from build123d import *

# Parameters (mm, degrees)
F2_DEPTH = 545


with BuildPart() as f2:
    # F0 (on Front) → F2 (new body)
    with BuildSketch(Plane.XZ):
        with BuildLine():
            Line((5.0927712857, 0), (1.5, 0))
            ThreePointArc((1.5, 0), (0.4393398282, -0.4393398282), (0, -1.5))
            Line((0, -1.5), (0, -5.0927712857))
            ThreePointArc((0, -5.0927712857), (0.0601351693, -5.3950911973), (0.2313856429, -5.6513856429))
            Line((0.2313856429, -5.6513856429), (1.69, -7.11))
            Line((1.69, -7.11), (1.8, -7.11))
            Line((1.8, -7.11), (1.8, -4.5006601718))
            Line((1.8, -4.5006601718), (3.44, -4.5006601718))
            Line((3.44, -4.5006601718), (6.1000000155, -7.1606601718))
            Line((6.1000000155, -7.1606601718), (6.1000000155, -9.9))
            Line((6.1000000155, -9.9), (6.2000000155, -10))
            Line((6.2000000155, -10), (6.1000000155, -10.1))
            Line((6.1000000155, -10.1), (6.1000000155, -12.8393398605))
            Line((6.1000000155, -12.8393398605), (3.44, -15.4993398916))
            Line((3.44, -15.4993398916), (1.8, -15.4993398916))
            Line((1.8, -15.4993398916), (1.8, -12.8893398916))
            Line((1.8, -12.8893398916), (1.69, -12.8893398916))
            Line((1.69, -12.8893398916), (0.2313856429, -14.3479542487))
            ThreePointArc((0.2313856429, -14.3479542487), (0.0601351693, -14.6042486943), (0, -14.9065686059))
            Line((0, -14.9065686059), (0, -20))
            Line((0, -20), (0, -25.0934313941))
            ThreePointArc((0, -25.0934313941), (0.0601351693, -25.3957513057), (0.2313856429, -25.6520457513))
            Line((0.2313856429, -25.6520457513), (1.69, -27.1106601084))
            Line((1.69, -27.1106601084), (1.8, -27.1106601084))
            Line((1.8, -27.1106601084), (1.8, -24.5006601084))
            Line((1.8, -24.5006601084), (3.44, -24.5006601084))
            Line((3.44, -24.5006601084), (6.1000000155, -27.1606601395))
            Line((6.1000000155, -27.1606601395), (6.1000000155, -29.9))
            Line((6.1000000155, -29.9), (6.2000000155, -30))
            Line((6.2000000155, -30), (6.1000000155, -30.1))
            Line((6.1000000155, -30.1), (6.1000000155, -32.8393398282))
            Line((6.1000000155, -32.8393398282), (3.44, -35.4993398282))
            Line((3.44, -35.4993398282), (1.8, -35.4993398282))
            Line((1.8, -35.4993398282), (1.8, -32.89))
            Line((1.8, -32.89), (1.69, -32.89))
            Line((1.69, -32.89), (0.2313856429, -34.3486143571))
            ThreePointArc((0.2313856429, -34.3486143571), (0.0601351693, -34.6049088027), (0, -34.9072287143))
            Line((0, -34.9072287143), (0, -38.5))
            ThreePointArc((0, -38.5), (0.4393398282, -39.5606601718), (1.5, -40))
            Line((1.5, -40), (5.0927712857, -40))
            ThreePointArc((5.0927712857, -40), (5.3950911973, -39.9398648307), (5.6513856429, -39.7686143571))
            Line((5.6513856429, -39.7686143571), (7.11, -38.31))
            Line((7.11, -38.31), (7.11, -38.2))
            Line((7.11, -38.2), (4.5006601718, -38.2))
            Line((4.5006601718, -38.2), (4.5006601718, -36.56))
            Line((4.5006601718, -36.56), (7.1606601873, -33.9))
            Line((7.1606601873, -33.9), (9.9000000155, -33.9))
            Line((9.9000000155, -33.9), (10.0000000478, -33.8000000323))
            Line((10.0000000478, -33.8000000323), (10.1000000802, -33.9))
            Line((10.1000000802, -33.9), (12.8393399084, -33.9))
            Line((12.8393399084, -33.9), (15.4993399239, -36.56))
            Line((15.4993399239, -36.56), (15.4993399239, -38.2))
            Line((15.4993399239, -38.2), (12.8900000957, -38.2))
            Line((12.8900000957, -38.2), (12.8900000957, -38.31))
            Line((12.8900000957, -38.31), (14.3486144528, -39.7686143571))
            ThreePointArc((14.3486144528, -39.7686143571), (14.6049088984, -39.9398648307), (14.90722881, -40))
            Line((14.90722881, -40), (18.5000000957, -40))
            ThreePointArc((18.5000000957, -40), (19.5606602675, -39.5606601718), (20.0000000957, -38.5))
            Line((20.0000000957, -38.5), (20.0000000957, -34.9072287143))
            ThreePointArc((20.0000000957, -34.9072287143), (19.9398649264, -34.6049088027), (19.7686144528, -34.3486143571))
            Line((19.7686144528, -34.3486143571), (18.3100000957, -32.89))
            Line((18.3100000957, -32.89), (18.2000000957, -32.89))
            Line((18.2000000957, -32.89), (18.2000000957, -35.4993398282))
            Line((18.2000000957, -35.4993398282), (16.5600000957, -35.4993398282))
            Line((16.5600000957, -35.4993398282), (13.9000000802, -32.8393398282))
            Line((13.9000000802, -32.8393398282), (13.9000000802, -30.1))
            Line((13.9000000802, -30.1), (13.8000000802, -30))
            Line((13.8000000802, -30), (13.9000000802, -29.9))
            Line((13.9000000802, -29.9), (13.9000000802, -27.1606601395))
            Line((13.9000000802, -27.1606601395), (16.5600000957, -24.5006601084))
            Line((16.5600000957, -24.5006601084), (18.2000000957, -24.5006601084))
            Line((18.2000000957, -24.5006601084), (18.2000000957, -27.1106601084))
            Line((18.2000000957, -27.1106601084), (18.3100000957, -27.1106601084))
            Line((18.3100000957, -27.1106601084), (19.7686144528, -25.6520457513))
            ThreePointArc((19.7686144528, -25.6520457513), (19.9398649264, -25.3957513057), (20.0000000957, -25.0934313941))
            Line((20.0000000957, -25.0934313941), (20.0000000957, -20))
            Line((20.0000000957, -20), (20.0000000957, -14.9065686059))
            ThreePointArc((20.0000000957, -14.9065686059), (19.9398649264, -14.6042486943), (19.7686144528, -14.3479542487))
            Line((19.7686144528, -14.3479542487), (18.3100000957, -12.8893398916))
            Line((18.3100000957, -12.8893398916), (18.2000000957, -12.8893398916))
            Line((18.2000000957, -12.8893398916), (18.2000000957, -15.4993398916))
            Line((18.2000000957, -15.4993398916), (16.5600000957, -15.4993398916))
            Line((16.5600000957, -15.4993398916), (13.9000000802, -12.8393398605))
            Line((13.9000000802, -12.8393398605), (13.9000000802, -10.1))
            Line((13.9000000802, -10.1), (13.8000000802, -10))
            Line((13.8000000802, -10), (13.9000000802, -9.9))
            Line((13.9000000802, -9.9), (13.9000000802, -7.1606601718))
            Line((13.9000000802, -7.1606601718), (16.5600000957, -4.5006601718))
            Line((16.5600000957, -4.5006601718), (18.2000000957, -4.5006601718))
            Line((18.2000000957, -4.5006601718), (18.2000000957, -7.11))
            Line((18.2000000957, -7.11), (18.3100000957, -7.11))
            Line((18.3100000957, -7.11), (19.7686144528, -5.6513856429))
            ThreePointArc((19.7686144528, -5.6513856429), (19.9398649264, -5.3950911973), (20.0000000957, -5.0927712857))
            Line((20.0000000957, -5.0927712857), (20.0000000957, -1.5))
            ThreePointArc((20.0000000957, -1.5), (19.5606602675, -0.4393398282), (18.5000000957, 0))
            Line((18.5000000957, 0), (14.90722881, 0))
            ThreePointArc((14.90722881, 0), (14.6049088984, -0.0601351693), (14.3486144528, -0.2313856429))
            Line((14.3486144528, -0.2313856429), (12.8900000957, -1.69))
            Line((12.8900000957, -1.69), (12.8900000957, -1.8))
            Line((12.8900000957, -1.8), (15.4993399239, -1.8))
            Line((15.4993399239, -1.8), (15.4993399239, -3.44))
            Line((15.4993399239, -3.44), (12.8393399084, -6.1))
            Line((12.8393399084, -6.1), (10.1000000802, -6.1))
            Line((10.1000000802, -6.1), (10.0000000478, -6.1999999677))
            Line((10.0000000478, -6.1999999677), (9.9000000155, -6.1))
            Line((9.9000000155, -6.1), (7.1606601873, -6.1))
            Line((7.1606601873, -6.1), (4.5006601718, -3.44))
            Line((4.5006601718, -3.44), (4.5006601718, -1.8))
            Line((4.5006601718, -1.8), (7.11, -1.8))
            Line((7.11, -1.8), (7.11, -1.69))
            Line((7.11, -1.69), (5.6513856429, -0.2313856429))
            ThreePointArc((5.6513856429, -0.2313856429), (5.3950911973, -0.0601351693), (5.0927712857, 0))
        make_face()
        Polygon((1.8, -38.2), (1.8, -36.57), (2.34, -36.57), (3.43, -37.66), (3.43, -38.2), align=None, mode=Mode.SUBTRACT)
        with BuildLine():
            ThreePointArc((10.0000000478, -27.9), (11.4849242883, -28.5150757595), (12.1000000478, -30))
            ThreePointArc((12.1000000478, -30), (11.4849242883, -31.4849242405), (10.0000000478, -32.1))
            ThreePointArc((10.0000000478, -32.1), (8.5150758074, -31.4849242405), (7.9000000478, -30))
            ThreePointArc((7.9000000478, -30), (8.5150758074, -28.5150757595), (10.0000000478, -27.9))
        make_face(mode=Mode.SUBTRACT)
        Polygon((17.6600000957, -36.57), (18.2000000957, -36.57), (18.2000000957, -38.2), (16.5700000957, -38.2), (16.5700000957, -37.66), align=None, mode=Mode.SUBTRACT)
        Polygon((9.9000000478, -13.9000000323), (10.0000000478, -13.8000000323), (10.1000000478, -13.9000000323), (12.8393399084, -13.9000000323), (16.2400000478, -17.3006601916), (18.2000000478, -17.3006601916), (18.2000000478, -20), (18.2000000478, -22.6993398084), (16.2400000478, -22.6993398084), (12.8393399084, -26.0999999677), (10.1000000478, -26.0999999677), (10.0000000478, -26.1999999677), (9.9000000478, -26.0999999677), (7.1606601873, -26.0999999677), (3.7600000478, -22.6993398084), (1.8000000478, -22.6993398084), (1.8000000478, -20), (1.8000000478, -17.3006601916), (3.7600000478, -17.3006601916), (7.1606601873, -13.9000000323), align=None, mode=Mode.SUBTRACT)
        Polygon((1.8, -3.43), (1.8, -1.8), (3.43, -1.8), (3.43, -2.34), (2.34, -3.43), align=None, mode=Mode.SUBTRACT)
        with BuildLine():
            ThreePointArc((7.9000000478, -10), (8.5150758074, -8.5150757595), (10.0000000478, -7.9))
            ThreePointArc((10.0000000478, -7.9), (11.4849242883, -8.5150757595), (12.1000000478, -10))
            ThreePointArc((12.1000000478, -10), (11.4849242883, -11.4849242405), (10.0000000478, -12.1))
            ThreePointArc((10.0000000478, -12.1), (8.5150758074, -11.4849242405), (7.9000000478, -10))
        make_face(mode=Mode.SUBTRACT)
        Polygon((16.5700000957, -2.34), (16.5700000957, -1.8), (18.2000000957, -1.8), (18.2000000957, -3.43), (17.6600000957, -3.43), align=None, mode=Mode.SUBTRACT)
    extrude(amount=F2_DEPTH)


solid = f2.part
CAD build for the part. Positions are in the model's coordinates, mm. Round coordinates to 2 decimals unless told otherwise and drop trailing zeros. Use a Markdown table: item, result. Add a question column.
1. Flat gauge pins, fed straight in: P1, Ø1, axis at x = 9, y = -232, coming from the +Z side; P2, Ø3, axis at x = 9, y = -161, coming from the -Z side; P3, Ø0.8, axis at y = -306.5, z = -9, coming from the +X side. Where does each tip first touch, or does it go through?
2. Slice it at A-A on y = -280.5. Give the number of separate pieces and of enclosed holes in the cut face, then the cut area to 3 significant figures.
3. Drill centre lines: probe 1 along X at (y, z) = (-508, -24); probe 2 along Z at (x, y) = (8.75, -132); probe 3 along Z at (x, y) = (13.5, -317). Where is each one in solid material? Low to high.
Reply:
| question | item | result |
|---|---|---|
| 1 | P1 | stops at z = -6.1 |
| 1 | P2 | stops at z = -33.9 |
| 1 | P3 | stops at x = 13.9 |
| 2 | separate pieces | 1 |
| 2 | enclosed holes | 7 |
| 2 | area | 291 mm^2 |
| 3 | probe 1 | x = 0 to 5.06, 14.94 to 20 |
| 3 | probe 2 | z = -33.9 to -31.69, -28.31 to -26.1, -13.9 to -11.69, -8.31 to -6.1 |
| 3 | probe 3 | z = -38.92 to -38.2, -34.56 to -25.44, -14.56 to -5.44, -1.8 to -1.08 |
